Autodesk Inventor part; units mm, degrees
ref_plane "YZ Plane" through (0, 0, 0) normal (1, 0, 0) x (0, 1, 0)
ref_plane "XZ Plane" through (0, 0, 0) normal (0, 1, 0) x (-1, 0, 0)
ref_plane "XY Plane" through (0, 0, 0) normal (0, 0, 1) x (1, 0, 0)
sketch "Sketch1" plane through (0, 0, 0) normal (0, 1, 0) x (-1, 0, 0)
  circle A0 centre (-20, 20) radius 2.5
  circle A1 centre (-20.0115, -20) radius 2.3331
  circle A2 centre (20, 20) radius 2.5
  circle A3 centre (19.9885, -20) radius 2.3169
  circle A4 centre (0, -0.053) radius 37.5
  line L0 (2.55, -7.239) -> (2.55, -9.7779)
  line L1 (2.55, -9.7779) -> (-2.55, -9.789)
  line L2 (-2.55, -9.789) -> (-2.55, -7.239)
  line L3 (-2.55, -5.5721) -> (2.55, -9.7779) construction
  line L4 (2.55, -5.561) -> (-2.55, -9.789) construction
  line L5 (0, -0.053) -> (0, -12.2317) construction
  arc A5 (2.55, -7.239) -> (-2.55, -7.239) centre (0, -0.053) ccw
  point P0 (0, 0)
  point P1 (0, -7.675)
  point P2 (2.55, -8.5084)
  point P3 (-2.55, -8.514)
  dimension "d1" = 40
  dimension "d2" = 40
  dimension "d3" = 40
  dimension "d4" = 40
  dimension "d10" = 75
  dimension "d16" = 0
  dimension "d17" = 2.55
  dimension "d19" = 5.1
  dimension "d20" = 0
  dimension "d21" = 0
  dimension "d22" = 2.1084
  dimension "d24" = 7.625
extrude "Extrusion1" add sketch "Sketch1" along normal blind 60
fillet "Fillet1" radius 0.5 4 edges at (37.5, 60, -0.053) (37.5, 0, -0.053) (0, 60, 7.572) (0, 0, 7.572)
fillet "Fillet2" radius 0.5 10 edges at (-2.55, 59.8545, -7.3953) (-2.55, 60, -8.7727) (-2.55, 0.1455, -7.3953) (-2.55, 0, -8.7727) (-2.55, 30, -7.239) (2.55, 59.8545, -7.3953) (2.55, 60, -8.7783) (2.55, 0.1455, -7.3953) (2.55, 0, -8.7783) (2.55, 30, -7.239)
properties part number "Flansch 3Ddruck"
The listing builds one solid part. Answer for the finished solid, in the listing's coordinates (mm). A direction names the side the tool comes from. Give positions to 0.01 mm unless a question says otherwise; leave off trailing zeros. Write each loop counter-clockwise with the first axis right and the second up, starting at its lowest first coordinate (ties: lowest second). Pieces come first, ordered by that corner, then holes.
1) A tool of negligible diameter and unlimited length cuts with its end or side. For faces 1 (the face through (1, 60, 9)), 2 (the face through (-2.55, 30, -9)), from which of +Z, -Z, +X, -X, +Y, -Y can it reach the whole face along a straight path? Write none if from no direction.
2) Section A-A (y = 48.5) is taken. Write down the section's boundary in (x, z).
3) Given P1, Ø3, axis at x = 4.5, y = 28, coming from the -Z side; P2, Ø5, axis at x = -5.5, y = 52.5, coming from the +Z side; P3, Ø8, axis at x = 19, y = 33.5, coming from the -Z side; P4, Ø13.5, axis at x = 0, z = -0.053, coming from the -Y side, each flat-ended and moving along its own axis, determine where each tip first touches the part or whether it passes through.
4) Find the intervals of material crossed by L1, parallel to X at y = 16.5, z = 21; L2, parallel to Z at x = -18, y = 23; L3, parallel to X at y = 14.5, z = 22, in increasing order.
5) Section B-B (x = -20) is taken. Count the separate pieces of the cut face and the enclosed holes in it, and give its area (3 significant figures).
6) For a pull along Z with two mould halves and no side action, classify faces 3 (the face through (1, 0, 9)), 4 (the face through (2.55, 30, -9)), 5 (the face through (22.342, 29.58, -20.103)), 6 (the face through (4.882, 29.587, -37.234)) as pulls with the +Z half, pulls with the -Z half, needs draft (parallel to the pull), parting line crosses it, or undercut.
Response:
1. face 1: +Z, -Z, +X, -X, +Y
1. face 2: +Y, -Y
2. outline: circle Ø75 at (0, -0.05); hole circle Ø5 at (-20, 20); hole circle Ø4.63 at (-19.99, -20); hole (-2.86, -7.12) arc R0.5 cw to (-2.55, -7.58) - (-2.55, -9.78) - (2.55, -9.79) - (2.55, -7.58) arc R0.5 cw to (2.86, -7.12) arc R7.63 ccw (long way) to start; hole circle Ø5 at (20, 20); hole circle Ø4.67 at (20.01, -20)
3. P1: stops at z = -37.43
3. P2: stops at z = 37.33
3. P3: stops at z = -34.42
3. P4: passes through
4. L1: x = -31.03 to -22.29, -17.71 to 17.71, 22.29 to 31.03
4. L2: z = -32.95 to -21.19, -18.81 to 18.5, 21.5 to 32.84
4. L3: x = -30.33 to -21.5, -18.5 to 18.5, 21.5 to 30.33
5. separate pieces: 3
5. enclosed holes: 0
5. area: 3,230 mm2
6. face 3: needs draft
6. face 4: undercut
6. face 5: undercut
6. face 6: parting line crosses it
